from build123d import *

# Parameters (mm, degrees)
F0_W     = 12
F0_H     = 15
F0_W_2   = 3
F1_DEPTH = 5
F2_DEPTH = 3
F3_W     = 15
F3_H     = 15
F3_R     = 2
F4_DEPTH = 8
F0_W_3   = 15
F0_R     = 2.025
F5_DEPTH = 5


# Not quite as in the source:
# - a feature names something its author has since deleted; it is built from what else it names


with BuildPart() as f1:
    # F0 (on Top) → F1 (new body)
    with BuildSketch(Plane.XY):
        with Locations((-9, -7.5)):
            Rectangle(F0_W, F0_H)
        with Locations((-1.5, -7.5)):
            Rectangle(F0_W_2, F0_H)
        Polygon((-3, 3), (-3, 0), (0, 0), (15, 0), (15, 3), align=None)
    extrude(amount=F1_DEPTH)

    # F0 (on Top) → F2 (join)
    with BuildSketch(Plane.XY):
        with Locations((-1.5, -7.5)):
            Rectangle(F0_W_2, F0_H)
        Polygon((-3, 3), (-3, 0), (0, 0), (15, 0), (15, 3), align=None)
    extrude(amount=-F2_DEPTH)

    # F3 (on face) → F4 (join)
    with BuildSketch(Plane(origin=(0, 0, -3), x_dir=(1, 0, 0), z_dir=(0, 0, -1))):
        with Locations((7.5, 7.5)):
            Rectangle(F3_W, F3_H)
        with Locations((7.5, 7.5)):
            Circle(F3_R, mode=Mode.SUBTRACT)
    extrude(amount=-F4_DEPTH)

    # F0 (on Top) → F5 (join)
    with BuildSketch(Plane.XY):
        with Locations((-22.5, -7.5)):
            Rectangle(F0_W_3, F0_H)
        with Locations((-22.5, -7.5)):
            Circle(F0_R, mode=Mode.SUBTRACT)
        with Locations((-22.5, 7.5)):
            Rectangle(F0_W_3, F0_H)
        Polygon((0, 15), (-15, 15), (-15, 0), (-3, 0), (-3, 3), (15, 3), (15, 15), align=None)
        with Locations((-7.5, 22.5)):
            Rectangle(F0_W_3, F0_H)
        with Locations((7.5, 22.5)):
            Rectangle(F0_W_3, F0_H)
        with Locations((7.5, 22.5)):
            Circle(F0_R, mode=Mode.SUBTRACT)
        with Locations((-22.5, 22.5)):
            Rectangle(F0_W_3, F0_H)
        with Locations((-22.5, 22.5)):
            Circle(F0_R, mode=Mode.SUBTRACT)
    extrude(amount=F5_DEPTH)


solid = f1.part
Can you work these out from the model? Positions are in its coordinate system, mm. A direction names the side the tool comes from. Coordinates: 2 decimals unless noted, no trailing zeros. Order: outer loops, then holes, each group sorted by start corner. A loop starts at its lowest first (then second) coordinate and runs counter-clockwise, first axis right, second up. Notation, with made-up numbers: (67.25, 56) - (78.25, 56) arc R24 cw to (78.25, 94) - close; hole circle Ø4 at (84, 60.25). An arc over 180 degrees is marked (long way). Answer as a JSON object with one key per item and string values. Group by question number.
Q1. On a 3-axis mill with a long thin cutter (end or side, diameter ignored), from which of +Z, -Z, +X, -X, +Y, -Y can I reach the whole of each face in a straight line? I mean faces 1 (the face through (-24.11, -8.73, 2.46)), 2 (the face through (6, 3, -1)). Say none if no direction works.
Q2. Imagine slicing it at C-C (z = 2.75). Please give me the cut outline in (x, y) (3 decimals), and give its area (3 significant figures).
Q3. Imagine slicing it at D-D (x = 7.5). Please give me the cut outline in (y, z) (3 decimals).
Q4. Imagine slicing it at A-A (y = 22.5). Please give me the cut outline in (x, z) (3 decimals).
Q5. Imagine slicing it at B-B (x = -22.5). Please give me the cut outline in (y, z) (3 decimals), and give its area (4 significant figures).
Q6. I need wall thicknesses on line 1 (Y direction, x = -22.5, z = 2.6) (3 decimals); line 2 (Y direction, x = 7.5, z = -0.25); line 3 (X direction, y = -7, z = 0.75). Which ranges of each line are inside material? Lowest first, please. Write a range as from..to.
Q7. Will these pins go through, and if not, where does the flat tip stop? P1, Ø1.5, axis at x = 6.5, z = -1.5, coming from the +Y side; P2, Ø3, axis at x = -22.5, y = 22.5, coming from the -Z side; P3, Ø5, axis at x = -11, y = 3, coming from the -Z side; P4, Ø2.5, axis at y = -2.5, z = -1.5, coming from the -X side.
Q8. We'd pull the mould along X, two halves only. Please class faces 3 (the face through (7.24, 24.51, 2.46)), 4 (the face through (-3, -6, -1)), 5 (the face through (-23.99, 23.87, 2.46)), 6 (the face through (-8, 8, 5)): +X half, -X half, draft (parallel to the pull), parting line (faces both ways), or undercut.
Determined:
{
 "1": {"face 1": "+Z, -Z", "face 2": "-Z, +X, -X, +Y"},
 "2": {"outline": "(-30, -15) - (15, -15) - (15, 30) - (-30, 30) - close; hole circle Ø4.05 at (-22.5, -7.5); hole circle Ø4.05 at (-22.5, 22.5); hole circle Ø4.05 at (7.5, 22.5); hole circle Ø4 at (7.5, -7.5)", "area": "1,970 mm2"},
 "3": {"outline": "(-15, -3) - (-9.5, -3) - (-9.5, 5) - (-15, 5) - close; (-5.5, -3) - (3, -3) - (3, 0) - (20.475, 0) - (20.475, 5) - (-5.5, 5) - close; (24.525, 0) - (30, 0) - (30, 5) - (24.525, 5) - close"},
 "4": {"outline": "(-30, 0) - (-24.525, 0) - (-24.525, 5) - (-30, 5) - close; (-20.475, 0) - (5.475, 0) - (5.475, 5) - (-20.475, 5) - close; (9.525, 0) - (15, 0) - (15, 5) - (9.525, 5) - close"},
 "5": {"outline": "(-15, 0) - (-9.525, 0) - (-9.525, 5) - (-15, 5) - close; (-5.475, 0) - (20.475, 0) - (20.475, 5) - (-5.475, 5) - close; (24.525, 0) - (30, 0) - (30, 5) - (24.525, 5) - close", "area": "184.5 mm2"},
 "6": {"line 1": "y = -15..-9.525, -5.475..20.475, 24.525..30", "line 2": "y = -15..-9.5, -5.5..3", "line 3": "x = -30..-24.46, -20.54..5.56, 9.44..15"},
 "7": {"P1": "stops at y = 3", "P2": "passes through", "P3": "stops at z = 0", "P4": "stops at x = -3"},
 "8": {"face 3": "undercut", "face 4": "-X half", "face 5": "undercut", "face 6": "draft"}
}
